Autodesk Inventor part; units mm, degrees
ref_plane "Work Plane2" through (32.194, 0, 0) normal (1, 0, 0) x (0, 1, 0)
ref_plane "XZ Plane" through (0, 0, 0) normal (0, 1, 0) x (-1, 0, 0)
ref_plane "XY Plane" through (0, 0, 0) normal (0, 0, 1) x (1, 0, 0)
sketch "Sketch1" plane through (0, 0, 0) normal (0, 0, 1) x (1, 0, 0)
  line L0 (0.2085, 0) -> (9, 0)
  line L1 (2.2118, 14.0222) -> (2.2118, 13.8222)
  line L2 (2.2118, 13.8222) -> (5.2118, 13.8222)
  line L3 (5.2118, 13.8222) -> (5.2118, 14.0222)
  line L4 (0.2118, 14) -> (2.2118, 14.0222)
  line L5 (5.2118, 14.0222) -> (32.2118, 14.5)
  line L6 (-8.963, 9) -> (0.2118, 14)
  line L7 (-8.963, 9) -> (-33.963, 9)
  line L8 (-33.963, 9) -> (-33.963, 11)
  line L9 (-33.963, 11) -> (-8.963, 11.25)
  line L10 (-8.963, 11.25) -> (0.2118, 16.2105)
  line L11 (0.2118, 16.2105) -> (32.1937, 16.5)
  line L12 (32.1937, 16.5) -> (32.2118, 14.5)
  point P0 (0, 0)
  dimension "d1" = 14.5
  dimension "d2" = 14
  dimension "d5" = 32
  dimension "d7" = 3
  dimension "d8" = 2
  dimension "d9" = 0.2
  dimension "d10" = 0.2
  dimension "d11" = 9
  dimension "d12" = 0
  dimension "d16" = 0
  dimension "d17" = 25
  dimension "d18" = 11.25
  dimension "d19" = 11
  dimension "d20" = 0
  dimension "d21" = 2
  dimension "d23" = 25
revolve "Revolution1" add sketch "Sketch1" angle 360 about axis through (0.2085, 0, 0) along (1, 0, 0)
ref_plane "Work Plane1" through (35, 0, 0) normal (1, 0, 0) x (0, 1, 0)
sketch "Sketch2" plane through (35, 0, 0) normal (1, 0, 0) x (0, 1, 0)
  circle A0 centre (0, 0) radius 16.5
  circle A1 centre (0, 0) radius 14.5
  line L0 (11.5082, -6) -> (14.5, -6)
  line L1 (14.5, -6) -> (14.5, 6)
  line L2 (14.5, 6) -> (11.5082, 6)
  line L3 (11.5082, 6) -> (11.5082, -6)
  line L4 (14.695, 6) -> (14.695, -6)
  line L5 (14.695, -6) -> (14.5, -6)
  line L6 (14.695, 6) -> (14.5, 6)
  dimension "d25" = 12
  dimension "d26" = 6
extrude "Extrusion1" cut sketch "Sketch2" against normal blind 6.788 contours A1 L0 L3 L2 | L1 L0 A1 | A1 L2 L1 picked at (12.5055, 0)
sketch "Sketch3" plane through (35, 0, 0) normal (1, 0, 0) x (0, 1, 0)
  point P0 (0, 0)
ref_plane "Work Plane2" through (32.194, 0, 0) normal (1, 0, 0) x (0, 1, 0)
equation "\"d10\" = d9"
properties part number "fitting non rebreathing valve v2"
Could you check a few things on this model? Use its own coordinates, in mm. A direction names the side the tool comes from. Give positions to 0.01 mm unless a question says otherwise; leave off trailing zeros. Order: outer loops, then holes, each group sorted by start corner. A loop starts at its lowest first (then second) coordinate and runs counter-clockwise, first axis right, second up. Notation, with made-up numbers: (-29.75, 52) - (26.25, 52) arc R23 ccw to (26.25, 62) - close; hole circle Ø9 at (-33, 82). An arc over 180 degrees is marked (long way). One line per item, written item: value. Start each with the question number.
1. For P1, Ø10, axis at x = -25, y = 2, coming from the -Z side; P2, Ø5, axis at x = -18, z = -2, coming from the +Y side; P3, Ø1, axis at x = 6, y = -11.5, coming from the +Z side, each with a flat end and sliding along its axis, tell me the tip position at first contact or that it passes through.
2. For faces 1 (the face through (-21.638, -1.172, -8.923)), 2 (the face through (-21.29, -8.83, -6.77)), 3 (the face through (30, 14, -6)), which set-ups out of +Z, -Z, +X, -X, +Y, -Y let a thin tool reach every point of the face, with its end or its side?
3. Imagine slicing it at B-B on x = -24.5. List the corners of the cut face in (y, z) for me.
4. Imagine slicing it at A-A on x = 8. List the corners of the cut face in (y, z) for me.
5. If I drill on probe 1 along Z at (x, y) = (3, 0); probe 2 along Z at (x, y) = (28.5, -1); probe 3 along Y at (x, z) = (-22.5, -7), over which ranges is the centre line in solid material (lowest first)?
6. Thinking about a two-plate mould opening in X: for faces 4 (the face through (30, 14.5, 0)), 5 (the face through (-33.963, 2, -9)), 6 (the face through (18.9, -14.25, 0.63)), 7 (the face through (1, -1.82, 13.89)), which applies, +X half, -X half, draft (parallel to the pull), parting line (faces both ways), or undercut?
Values:
1. P1: z = -11.14
1. P2: y = 11.18
1. P3: z = 11.98
2. face 1: +X, -X
2. face 2: -X
2. face 3: +X
3. outline: circle Ø22.19 at (0, 0); hole circle Ø18 at (0, 0)
4. outline: circle Ø32.56 at (0, 0); hole circle Ø28.14 at (0, 0)
5. probe 1: -16.24 to -13.82, 13.82 to 16.24
5. probe 2: -16.44 to -14.4, 14.4 to 16.44
5. probe 3: -8.63 to -5.66, 5.66 to 8.63
6. face 4: draft
6. face 5: -X half
6. face 6: +X half
6. face 7: undercut
